Autodesk Inventor part; units mm, degrees
ref_plane "YZ Plane" through (0, 0, 0) normal (1, 0, 0) x (0, 1, 0)
ref_plane "XZ Plane" through (0, 0, 0) normal (0, 1, 0) x (-1, 0, 0)
ref_plane "XY Plane" through (0, 0, 0) normal (0, 0, 1) x (1, 0, 0)
sketch "Sketch1" plane through (0, 0, 0) normal (0, 1, 0) x (-1, 0, 0)
  line L0 (2.5, 0) -> (62.5, 0)
  line L1 (65, 37.5) -> (65, 53.5)
  line L2 (62.5, 56) -> (2.5, 56)
  line L3 (0, 53.5) -> (0, 2.5)
  line L4 (64.5, 37) -> (63, 37)
  line L5 (62.5, 36.5) -> (62.5, 19.5)
  line L6 (63, 19) -> (64.5, 19)
  line L7 (62.5, 37) -> (62.5, 56) construction
  line L8 (62.5, 19) -> (62.5, 0) construction
  arc A0 (65, 53.5) -> (62.5, 56) centre (62.5, 53.5) ccw
  arc A1 (62.5, 0) -> (65, 2.5) centre (62.5, 2.5) ccw
  arc A2 (0, 2.5) -> (2.5, 0) centre (2.5, 2.5) ccw
  arc A3 (2.5, 56) -> (0, 53.5) centre (2.5, 53.5) ccw
  arc A4 (64.5, 37) -> (65, 37.5) centre (64.5, 37.5) ccw
  arc A5 (63, 37) -> (62.5, 36.5) centre (63, 36.5) ccw
  arc A6 (62.5, 19.5) -> (63, 19) centre (63, 19.5) ccw
  line L9 (65, 18.5) -> (65, 2.5)
  arc A7 (65, 18.5) -> (64.5, 19) centre (64.5, 18.5) ccw
  line L10 (59, 0) -> (6, 0)
  line L11 (6, -0.5) -> (6, 8)
  line L12 (6, 8) -> (59, 8)
  line L13 (59, 8) -> (59, -0.5)
  line L14 (59, 8) -> (65, 8) construction
  line L15 (6, 8) -> (0, 8) construction
  line L16 (65.5, 53.5) -> (65.5, 37.5)
  arc A8 (64.5, 36.5) -> (65.5, 37.5) centre (64.5, 37.5) ccw
  line L17 (64.5, 36.5) -> (63, 36.5)
  line L18 (63, 36.5) -> (63, 19.5)
  line L19 (63, 19.5) -> (64.5, 19.5)
  arc A9 (65.5, 18.5) -> (64.5, 19.5) centre (64.5, 18.5) ccw
  line L20 (65.5, 18.5) -> (65.5, 2.5)
  arc A10 (62.5, -0.5) -> (65.5, 2.5) centre (62.5, 2.5) ccw
  line L21 (62.5, -0.5) -> (2.5, -0.5)
  arc A11 (-0.5, 2.5) -> (2.5, -0.5) centre (2.5, 2.5) ccw
  line L22 (-0.5, 2.5) -> (-0.5, 53.5)
  arc A12 (2.5, 56.5) -> (-0.5, 53.5) centre (2.5, 53.5) ccw
  line L23 (2.5, 56.5) -> (62.5, 56.5)
  arc A13 (65.5, 53.5) -> (62.5, 56.5) centre (62.5, 53.5) ccw
  line L24 (65.5, 37.5) -> (65.5, 18.5)
  point P0 (0, 0)
  point P1 (65, 56)
  point P2 (65, 0)
  point P3 (0, 56)
  point P4 (65, 19)
  dimension "d0" = 65
  dimension "d1" = 56
  dimension "d2" = 2.5
  dimension "d3" = 18
  dimension "d4" = 2.5
  dimension "d5" = 0.5
  dimension "d6" = 0.5
  dimension "d7" = 53
  dimension "d9" = 0.5
  dimension "d10" = 8
extrude "Extrusion1" add sketch "Sketch1" along normal blind 4 contours A2 L3 A3 L2 A0 L1 A4 L4 A5 L5 A6 L6 A7 L9 A1 L0 L13 L12 L11 | L0 L11 L21 A11 L22 A12 L23 A13 L16 A8 L17 L18 L19 A9 L20 A10 L13 A1 L9 A7 L6 A6 L5 A5 L4 A4 L1 A0 L2 A3 L3 A2 | A9 L19 L18 L17 A8 L24
sketch "Sketch2" plane through (0, 4, 0) normal (0, 1, 0) x (1, 0, 0)
  line L0 (-61.5, -52.5) -> (-3.5, -52.5) construction
  line L1 (-3.5, -52.5) -> (-3.5, -3.5) construction
  line L2 (-3.5, -3.5) -> (-61.5, -3.5) construction
  line L3 (-61.5, -3.5) -> (-61.5, -52.5) construction
  line L4 (-65.5, -2.5) -> (-65.5, -53.5) construction
  arc A0 (-65.5, -53.5) -> (-62.5, -56.5) centre (-62.5, -53.5) ccw construction
  line L5 (-62.5, -56.5) -> (-2.5, -56.5) construction
  arc A1 (-2.5, -56.5) -> (0.5, -53.5) centre (-2.5, -53.5) ccw construction
  line L6 (0.5, -53.5) -> (0.5, -2.5) construction
  arc A2 (0.5, -2.5) -> (-2.5, 0.5) centre (-2.5, -2.5) ccw construction
  line L7 (-2.5, 0.5) -> (-6, 0.5) construction
  line L8 (-6, 0.5) -> (-6, -8) construction
  line L9 (-6, -8) -> (-59, -8) construction
  line L10 (-59, -8) -> (-59, 0.5) construction
  line L11 (-59, 0.5) -> (-62.5, 0.5) construction
  arc A3 (-62.5, 0.5) -> (-65.5, -2.5) centre (-62.5, -2.5) ccw construction
  line L12 (-61.5, -28) -> (-65.5, -28) construction
  line L13 (-65.5, -2.5) -> (-65.5, -53.5) construction
  line L14 (-32.5, -52.5) -> (-32.5, -56.5) construction
  line L15 (-62.5, -56.5) -> (-2.5, -56.5) construction
  line L16 (-3.5, -26.1525) -> (0.5, -26.1525) construction
  line L17 (0.5, -53.5) -> (0.5, -2.5) construction
  line L18 (-5.4848, -3.5) -> (-5.4848, 0.5) construction
  line L19 (-2.5, 0.5) -> (-6, 0.5) construction
  circle A4 centre (-61.5, -52.5) radius 1.1
  circle A5 centre (-61.5, -3.5) radius 1.1
  circle A6 centre (-3.5, -52.5) radius 1.1
  circle A7 centre (-3.5, -3.5) radius 1.1
  circle A8 centre (-61.5, -52.5) radius 2.5
  circle A9 centre (-61.5, -3.5) radius 2.5
  circle A10 centre (-3.5, -3.5) radius 2.5
  circle A11 centre (-3.5, -52.5) radius 2.5
  point P0 (0, 0)
  dimension "d13" = 58
  dimension "d14" = 49
  dimension "d15" = 2.2
  dimension "d16" = 2.2
  dimension "d17" = 2.2
  dimension "d18" = 2.2
  dimension "d19" = 5
  dimension "d20" = 5
  dimension "d21" = 5
  dimension "d22" = 5
extrude "Extrusion2" add sketch "Sketch2" along normal blind 3
sketch "Sketch3" plane through (-3.5, 4, 3.5) normal (0, 1, 0) x (1, 0, 0)
  circle A0 centre (0, 0) radius 1.1
  circle A1 centre (0, -49) radius 1.1
  circle A2 centre (-58, -49) radius 1.1
  circle A3 centre (-58, 0) radius 1.1
  point P0 (3.5, 3.5)
extrude "Extrusion3" cut sketch "Sketch3" against normal blind 4
sketch "Sketch4" plane through (0, 0, 0) normal (0, -1, 0) x (1, 0, 0)
  circle A0 centre (-61.5, 52.5) radius 1.1
  circle A1 centre (-3.5, 52.5) radius 1.1
  circle A2 centre (-61.5, 3.5) radius 1.1
  circle A3 centre (-3.5, 3.5) radius 1.1
  line L0 (-65.5, 2.5) -> (-65.5, 53.5)
  arc A4 (-65.5, 2.5) -> (-62.5, -0.5) centre (-62.5, 2.5) ccw
  line L1 (-59, -0.5) -> (-62.5, -0.5)
  line L2 (-59, 8) -> (-59, -0.5)
  line L3 (-6, 8) -> (-59, 8)
  line L4 (-6, -0.5) -> (-6, 8)
  line L5 (-2.5, -0.5) -> (-6, -0.5)
  arc A5 (-2.5, -0.5) -> (0.5, 2.5) centre (-2.5, 2.5) ccw
  line L6 (0.5, 53.5) -> (0.5, 2.5)
  arc A6 (0.5, 53.5) -> (-2.5, 56.5) centre (-2.5, 53.5) ccw
  line L7 (-62.5, 56.5) -> (-2.5, 56.5)
  arc A7 (-62.5, 56.5) -> (-65.5, 53.5) centre (-62.5, 53.5) ccw
  line L8 (-68.5, 53.5) -> (-68.5, 2.5)
  arc A8 (-68.5, 2.5) -> (-62.5, -3.5) centre (-62.5, 2.5) ccw
  line L9 (-62.5, -3.5) -> (-56, -3.5)
  line L10 (-56, -3.5) -> (-56, 5)
  line L11 (-56, 5) -> (-9, 5)
  line L12 (-9, 5) -> (-9, -3.5)
  line L13 (-9, -3.5) -> (-2.5, -3.5)
  arc A9 (-2.5, -3.5) -> (3.5, 2.5) centre (-2.5, 2.5) ccw
  line L14 (3.5, 2.5) -> (3.5, 53.5)
  arc A10 (3.5, 53.5) -> (-2.5, 59.5) centre (-2.5, 53.5) ccw
  line L15 (-2.5, 59.5) -> (-62.5, 59.5)
  arc A11 (-62.5, 59.5) -> (-68.5, 53.5) centre (-62.5, 53.5) ccw
  line L16 (-67.6962, -0.5) -> (2.6962, -0.5)
  point P0 (0, 0)
  point P1 (-62.5, -0.5)
  dimension "d27" = 3
extrude "Extrusion4" add sketch "Sketch4" against normal blind 8.65 contours A4 L16 A8 L8 A11 L15 A10 L14 A9 A5 L6 A6 L7 A7 L0
sketch "Sketch5" plane through (0, 0, 0) normal (0, -1, 0) x (1, 0, 0)
  circle A0 centre (-61.5, 52.5) radius 1.1
  circle A1 centre (-3.5, 52.5) radius 1.1
  circle A2 centre (-61.5, 3.5) radius 1.1
  circle A3 centre (-3.5, 3.5) radius 1.1
  line L0 (-6, -0.5) -> (2.6962, -0.5)
  arc A4 (2.6962, -0.5) -> (3.5, 2.5) centre (-2.5, 2.5) ccw
  line L1 (3.5, 2.5) -> (3.5, 53.5)
  arc A5 (3.5, 53.5) -> (-2.5, 59.5) centre (-2.5, 53.5) ccw
  line L2 (-2.5, 59.5) -> (-62.5, 59.5)
  arc A6 (-62.5, 59.5) -> (-68.5, 53.5) centre (-62.5, 53.5) ccw
  line L3 (-68.5, 53.5) -> (-68.5, 2.5)
  arc A7 (-68.5, 2.5) -> (-67.6962, -0.5) centre (-62.5, 2.5) ccw
  line L4 (-59, -0.5) -> (-67.6962, -0.5)
  line L5 (-59, 8) -> (-59, -0.5)
  line L6 (-6, 8) -> (-59, 8)
  line L7 (-6, -0.5) -> (-6, 8)
  line L8 (-68.5, 53.5) -> (-68.5, 2.5)
  line L9 (-68.5, 9.5) -> (3.5, 9.5)
  line L10 (3.5, 53.5) -> (3.5, 2.5)
  point P0 (0, 0)
  point P1 (3.5, 9.5)
  dimension "d30" = 10
extrude "Extrusion5" add sketch "Sketch5" along normal blind 15 contours L9 L3 A6 L2 A5 L1
sketch "Sketch6" plane through (0, -15, 0) normal (0, -1, 0) x (1, 0, 0)
  line L0 (-82.5, -4.1741) -> (-82.5, 71.2939) construction
  line L1 (-62.5, 59.5) -> (-2.5, 59.5) construction
  line L2 (-82.5, 17) -> (-68.5, 17) construction
  line L3 (-68.5, 53.5) -> (-68.5, 9.5) construction
  line L4 (-82.5, 42) -> (-68.5, 42) construction
  line L5 (-75.5, 17) -> (-75.5, 42) construction
  line L6 (-6, -0.5) -> (2.6962, -0.5) construction
  circle A0 centre (-78.011, 17) radius 3
  arc A1 (-75.5, 24.0672) -> (-78.011, 9.5) centre (-78.011, 17) ccw
  line L7 (-68.5, 9.5) -> (-78.011, 9.5)
  line L8 (-68.5, 9.5) -> (3.5, 9.5)
  line L9 (-68.5, 24.5) -> (-78.011, 24.5)
  line L10 (-75.5, 29.5) -> (-82.5, 29.5) construction
  circle A2 centre (-78.011, 42) radius 3
  arc A3 (-78.011, 49.5) -> (-75.5, 34.9328) centre (-78.011, 42) ccw
  line L11 (-68.5, 49.5) -> (-78.011, 49.5)
  line L12 (-68.5, 34.5) -> (-78.011, 34.5)
  line L13 (-32.5, 59.5) -> (-32.5, 87.6423) construction
  circle A4 centre (13.011, 17) radius 3
  arc A5 (13.011, 9.5) -> (13.011, 24.5) centre (13.011, 17) ccw
  line L14 (3.5, 9.5) -> (13.011, 9.5)
  line L15 (3.5, 24.5) -> (13.011, 24.5)
  line L16 (3.5, 34.5) -> (13.011, 34.5)
  arc A6 (13.011, 34.5) -> (13.011, 49.5) centre (13.011, 42) ccw
  circle A7 centre (13.011, 42) radius 3
  line L17 (3.5, 49.5) -> (13.011, 49.5)
  line L18 (3.5, 53.5) -> (3.5, 2.5)
  line L19 (-68.5, 2.5) -> (-68.5, 53.5)
  point P0 (0, 0)
  point P1 (17.5, 17)
  point P2 (10.5, 17)
  point P3 (10.5, 42)
  dimension "d33" = 50
  dimension "d34" = 60
  dimension "d35" = 30
  dimension "d36" = 25
  dimension "d37" = 6
extrude "Extrusion6" add sketch "Sketch6" against normal blind 4
fillet "Fillet1" radius 1 4 edges at (-4.6, 7, 52.5) (-62.6, 7, 52.5) (-4.6, 7, 3.5) (-62.6, 7, 3.5)
equation "\"d5\" = d6"
equation "\"d16\" = d15"
equation "\"d17\" = d15"
equation "\"d18\" = d15"
equation "\"d20\" = d19"
equation "\"d21\" = d19"
equation "\"d22\" = d19"
equation "\"d35\" = 0.5 * d34"
properties part number "Pi GPIO Mount"
Model file for the job. Use its own axes, mm. A direction names the side the tool comes from. Round coordinates to 2 decimals unless told otherwise and drop trailing zeros. Loops run counter-clockwise (first coordinate to the right, second up) from the corner with the lowest first, then second, coordinate; pieces in that order, holes last.
1. Band-saw the part on A-A, the plane z = 42. List the corners of the cut face in (x, y), and give its area (3 significant figures).
Check values:
outline: (-85.51, -15) - (-81.01, -15) - (-81.01, -11) - (-85.51, -11) - close; (-75.01, -15) - (10.01, -15) - (10.01, -11) - (3.5, -11) - (3.5, 8.65) - (0.5, 8.65) - (0.5, 4) - (-65.5, 4) - (-65.5, 8.65) - (-68.5, 8.65) - (-68.5, -11) - (-75.01, -11) - close; (16.01, -15) - (20.51, -15) - (20.51, -11) - (16.01, -11) - close
area: 1,480 mm2
2. Band-saw the part on D-D, the plane x = -43. List the corners of the cut face in (y, z), and give its area (3 significant figures).
Check values:
outline: (-15, 9.5) - (0, 9.5) - (0, 8) - (4, 8) - (4, 56.5) - (8.65, 56.5) - (8.65, 59.5) - (-15, 59.5) - close
area: 970 mm2
3. Mould opens along Z. For faces 5 (the flat face through (0.5, 6, 28)), 6 (the flat face through (-73, -13, 49.5)), 7 (the cylindrical face through (3.29, 4.26, 0.93)) say: +Z half, -Z half, draft (parallel to the pull), parting line (faces both ways), or undercut.
Check values:
face 5: undercut
face 6: +Z half
face 7: -Z half
4. Drop flat-ended pins along their axis: P1, Ø3, axis at x = 6, y = -12, coming from the -Z side; P2, Ø7.5, axis at x = 13, z = 44.5, coming from the +Y side; P3, Ø5, axis at y = 6, z = 34.5, coming from the +X side. Give the stop position or say it passes through.
Check values:
P1: stops at z = 9.5
P2: stops at y = -11
P3: stops at x = 3.5
5. Band-saw the part on B-B, the plane x = -61.5. List the corners of the cut face in (y, z).
Check values:
outline: (-15, 9.5) - (0, 9.5) - (0, 4.6) - (6, 4.6) arc R1 ccw to (7, 5.6) - (7, 6) - (4, 6) - (4, 50) - (7, 50) - (7, 50.4) arc R1 ccw to (6, 51.4) - (-15, 51.4) - close; (-15, 53.6) - (6, 53.6) arc R1 ccw to (7, 54.6) - (7, 55) - (4, 55) - (4, 56.5) - (8.65, 56.5) - (8.65, 59.5) - (-15, 59.5) - close; (0, -0.5) - (4, -0.5) - (4, 1) - (7, 1) - (7, 1.4) arc R1 ccw to (6, 2.4) - (0, 2.4) - close
6. Tool access for faces 1 (the flat face through (8, -13, 24.5)), 2 (the flat face through (-73, -13, 24.5)), 3 (the cylindrical face through (-1.115, 5.479, 4.251)), 4 (the cylindrical face through (15.8, -13, 15.9)): list every direction of +Z, -Z, +X, -X, +Y, -Y with a clear straight run to the whole face (end or side of a thin tool).
Check values:
face 1: +X, +Y, -Y
face 2: -X, +Y, -Y
face 3: +Y
face 4: +Y, -Y
7. Wall check: probe 1 along Z at (x, y) = (-61.5, 2.5); probe 2 along Z at (x, y) = (-24, -8.75); probe 3 along Y at (x, z) = (-74.5, 42). Give the ranges that are in metal, low to high.
Check values:
probe 1: z = -0.5 to 2.4, 4.6 to 51.4, 53.6 to 59.5
probe 2: z = 9.5 to 59.5
probe 3: y = -15 to -11
8. Band-saw the part on C-C, the plane y = -7.5. List the corners of the cut face in (x, z), and give its area (3 significant figures).
Check values:
outline: (-68.5, 9.5) - (3.5, 9.5) - (3.5, 53.5) arc R6 ccw to (-2.5, 59.5) - (-62.5, 59.5) arc R6 ccw to (-68.5, 53.5) - close; hole circle Ø2.2 at (-61.5, 52.5); hole circle Ø2.2 at (-3.5, 52.5)
area: 3,580 mm2
